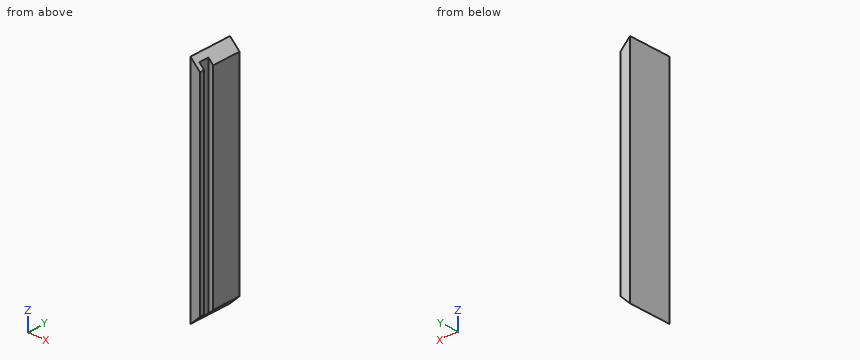
Autodesk Inventor part; units mm, degrees
ref_plane "YZ Plane" through (0, 0, 0) normal (1, 0, 0) x (0, 1, 0)
ref_plane "XZ Plane" through (0, 0, 0) normal (0, 1, 0) x (-1, 0, 0)
ref_plane "XY Plane" through (0, 0, 0) normal (0, 0, 1) x (1, 0, 0)
sketch "Sketch1" plane through (0, 0, 0) normal (0, 1, 0) x (-1, 0, 0)
  line L0 (0, 47) -> (0, -47)
  line L1 (-4, 43) -> (-4, -43)
  line L2 (0, 0) -> (-19.6483, 0) construction
  line L3 (-4, 43) -> (0, 47)
  line L4 (0, -47) -> (-4, -43)
  point P0 (-4, 0)
  dimension "d6" = 94
  dimension "d7" = 86
  dimension "d8" = 4
extrude "Extrusion1" add sketch "Sketch1" along normal blind 18
sketch "Sketch2" plane through (4, 0, 43) normal (1, 0, 0) x (0, 0, -1)
  line L0 (-4, 0) -> (-4, 18)
  line L1 (90, 0) -> (90, 18)
  line L2 (-4, 6) -> (90, 6)
  line L3 (90, 6) -> (90, 1.9)
  line L4 (90, 1.9) -> (-4, 1.9)
  line L5 (-4, 1.9) -> (-4, 6)
  line L6 (0, 0) -> (86, 0)
  point P0 (43, 0)
  point P1 (-4, 1.9)
  dimension "d11" = 4.1
  dimension "d12" = 1.9
extrude "Extrusion2" cut sketch "Sketch2" against normal blind 2
properties part number "long PDMS Chamber side"
Could you check a few things on this model? Use its own coordinates, in mm. Give positions to 0.01 mm unless a question says otherwise; leave off trailing zeros. Order: outer loops, then holes, each group sorted by start corner. A loop starts at its lowest first (then second) coordinate and runs counter-clockwise, first axis right, second up. Notation, with made-up numbers: (33.25, 84.25) - (75.25, 84.25) arc R21 cw to (75.25, 123.25) - close; hole circle Ø5 at (-20, 36). An arc over 180 degrees is marked (long way). One line per question, with ' | ' between items. Start each with the question number.
Item 1: I want a section at B-B on z = 21. Write out the boundary of the cut face in (x, y).
Item 2: I want a section at D-D on y = 12.5. Write out the boundary of the cut face in (x, z), then the cut area to 3 significant figures.
Item 3: I'm going to push flat-ended pins straight in: pin 1 Ø1.5 at (x, y) = (0.5, 3.5) entering from -Z; pin 2 Ø8 at (y, z) = (3.5, -19) entering from +X; pin 3 Ø3.5 at (y, z) = (4, -7.5) entering from +X. Where does each tip first touch, or does it pass through?
Item 4: I want a section at A-A on x = 2.7. Write out the boundary of the cut face in (y, z).
Item 5: I want a section at C-C on y = 4. Write out the boundary of the cut face in (x, z), then the cut area to 3 significant figures.
Item 6: I need wall thicknesses on probe 1 along Y at (x, z) = (2.1, -38); probe 2 along X at (y, z) = (4.25, 6); probe 3 along Z at (x, y) = (0.45, 1.75). Which ranges of each line are inside material? Lowest first, please. Write a range as [from, to].
Verdict:
1) outline: (0, 0) - (4, 0) - (4, 1.9) - (2, 1.9) - (2, 6) - (4, 6) - (4, 18) - (0, 18) - close
2) outline: (0, -47) - (4, -43) - (4, 43) - (0, 47) - close | area: 360 mm^2
3) pin 1: z = -47 | pin 2: x = 4 | pin 3: x = 2
4) outline: (0, -44.3) - (1.9, -44.3) - (1.9, 44.3) - (0, 44.3) - close; (6, -44.3) - (18, -44.3) - (18, 44.3) - (6, 44.3) - close
5) outline: (0, -47) - (2, -45) - (2, 45) - (0, 47) - close | area: 184 mm^2
6) probe 1: [0, 1.9], [6, 18] | probe 2: [0, 2] | probe 3: [-46.55, 46.55]
